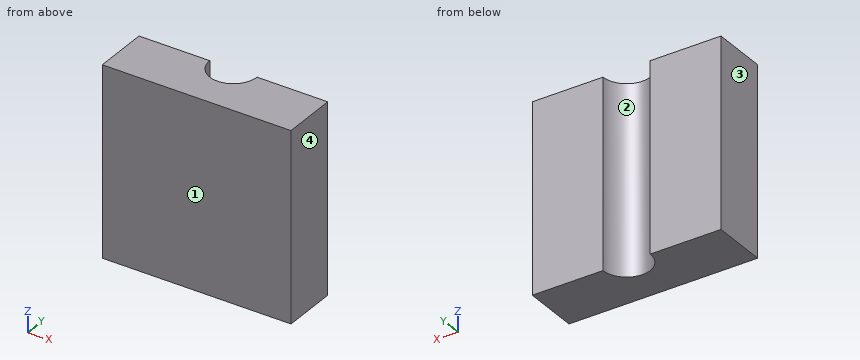
Autodesk Inventor part; units mm, degrees
ref_plane "YZ Plane" through (0, 0, 0) normal (1, 0, 0) x (0, 1, 0)
ref_plane "XZ Plane" through (0, 0, 0) normal (0, 1, 0) x (-1, 0, 0)
ref_plane "XY Plane" through (0, 0, 0) normal (0, 0, 1) x (1, 0, 0)
sketch "Sketch1" plane through (0, 0, 0) normal (0, 1, 0) x (-1, 0, 0)
  line L0 (-19.05, 19.05) -> (-19.05, -19.05)
  line L1 (-19.05, -19.05) -> (19.05, -19.05)
  line L2 (19.05, -19.05) -> (19.05, 19.05)
  line L3 (19.05, 19.05) -> (-19.05, 19.05)
  line L4 (-19.05, 19.05) -> (19.05, -19.05) construction
  line L5 (-19.05, -19.05) -> (19.05, 19.05) construction
  point P0 (0, 0)
  dimension "d0" = 38.1
extrude "Extrusion1" add sketch "Sketch1" along normal blind 11.1125
sketch "Sketch2" plane through (-19.05, 0, 19.05) normal (0, 0, 1) x (1, 0, 0)
  line L0 (38.1, 11.1125) -> (0, 11.1125)
  arc A0 (14.2875, 11.1125) -> (23.8125, 11.1125) centre (19.05, 11.1125) ccw
  point P0 (19.05, 0)
  dimension "d3" = 9.525
extrude "Extrusion2" cut sketch "Sketch2" against normal through all
equation "\"d0\" = width"
equation "\"d1\" = heightOfBottomHole"
equation "\"d3\" = bottomHoleDiam"
equation "\"d4\" = deltaBottomToTop"
equation "\"bottomHoleDiam\" = 9.525"
equation "\"width\" = 38.1"
equation "\"height\" = deltaBottomToTop + heightOfBottomHole + heightOfTopHole"
equation "\"deltaBottomToTop\" = 25.4"
properties part number "BottomOfSquareSupport"
Input: part model. Units: mm. Frame: model coordinates. Face numbers are marked on the shaded views. Round coordinates to 2 decimals unless told otherwise and drop trailing zeros. Order: outer loops, then holes, each group sorted by start corner. A loop starts at its lowest first (then second) coordinate and runs counter-clockwise, first axis right, second up. Notation, with made-up numbers: (-7, 71.25) - (17, 71.25) arc R18 ccw to (17, 87.25) - close; hole circle Ø11 at (62, 12.5). An arc over 180 degrees is marked (long way). One line per question, with ' | ' between items. Start each with the question number.
1) Pull-direction query (X, two-part tool) for the marked faces 1, 2, 3 and 4; classes: +X half, -X half, draft (parallel to the pull), parting line (faces both ways), or undercut.
2) Cut plane C-C, the plane x = 0. Return the cut outline in (y, z).
3) Ray query, probe 1 along X at (y, z) = (7, 7.5); probe 2 along X at (y, z) = (7.5, 6); probe 3 along Y at (x, z) = (-3, 3). Return the intervals inside material, ascending.
4) Cut plane B-B, the plane y = 9. Return the cut outline in (x, z).
Worked out:
1) face 1: draft | face 2: undercut | face 3: -X half | face 4: +X half
2) outline: (0, -19.05) - (6.35, -19.05) - (6.35, 19.05) - (0, 19.05) - close
3) probe 1: x = -19.05 to -2.4, 2.4 to 19.05 | probe 2: x = -19.05 to -3.1, 3.1 to 19.05 | probe 3: y = 0 to 7.41
4) outline: (-19.05, -19.05) - (-4.27, -19.05) - (-4.27, 19.05) - (-19.05, 19.05) - close; (4.27, -19.05) - (19.05, -19.05) - (19.05, 19.05) - (4.27, 19.05) - close
